Autodesk Inventor part; units mm, degrees
ref_plane "YZ Plane" through (0, 0, 0) normal (1, 0, 0) x (0, 1, 0)
ref_plane "XZ Plane" through (0, 0, 0) normal (0, 1, 0) x (-1, 0, 0)
ref_plane "XY Plane" through (0, 0, 0) normal (0, 0, 1) x (1, 0, 0)
sketch "Sketch1" plane through (0, 0, 0) normal (0, 1, 0) x (-1, 0, 0)
  circle A0 centre (0, 0) radius 15.875
  dimension "d7" = 31.75
extrude "Extrusion1" add sketch "Sketch1" along normal mid plane 159.2
sketch "Sketch2" plane through (0, 79.6, 0) normal (0, 1, 0) x (1, 0, 0)
  circle A0 centre (0, 0) radius 12.7
  circle A1 centre (0, 0) radius 15.875
  circle A2 centre (0, 0) radius 15.875
  dimension "d6" = 25.4
extrude "Extrusion2" cut sketch "Sketch2" against normal blind 54
fillet "Fillet1" radius 0.8 1 edges at (-12.7, 25.6, 0)
mirror "Mirror2" about plane through (0, -79.6, 0) normal (0, -1, 0) of "Extrusion2", "Extrusion1", "Fillet1"
properties part number "Eje Biela"
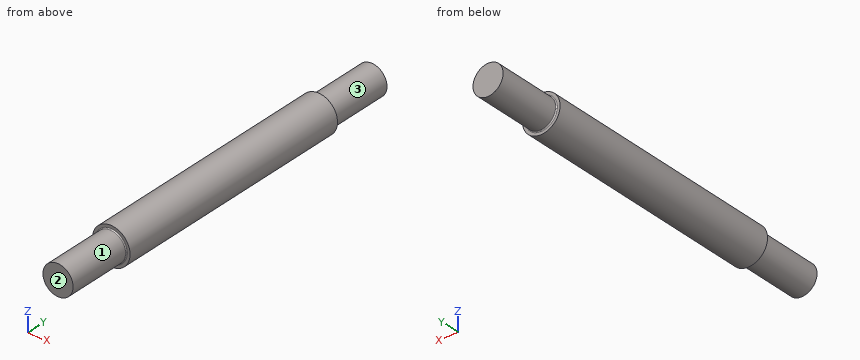
Build history of the part. All positions in model axes, mm. Face numbers are marked on the shaded views. A direction names the side the tool comes from. Give positions to 0.01 mm unless a question says otherwise; leave off trailing zeros. Write each loop counter-clockwise with the first axis right and the second up, starting at its lowest first coordinate (ties: lowest second). Pieces come first, ordered by that corner, then holes. Notation, with made-up numbers: (-17.75, 25) - (8.25, 25) arc R27 ccw to (8.25, 61) - close; hole circle Ø6 at (33, 31.5). An arc over 180 degrees is marked (long way). Use one line per item in the form item = value. Start each with the question number.
1. Band-saw the part on A-A on x = 0. Write the cut outline in (y, z) (3 decimals), plus the area to 3 significant figures.
2. Band-saw the part on C-C on y = -198.5. Write the cut outline in (x, z).
3. Band-saw the part on D-D on y = -149. Write the cut outline in (x, z) (3 decimals).
4. 3-axis set-ups, long thin cutter, end or side, ignore diameter. For the marked faces 1, 2 and 3: which of +Z, -Z, +X, -X, +Y, -Y reach the whole face in a straight line?
5. Probe line 1 (Z direction, x = -1, y = -197); line 2 (Y direction, x = -14, z = -5); line 3 (X direction, y = -84.5, z = 11). List the from-to ranges inside material, lowest first. Write a range as [from, to].
6. Band-saw the part on B-B on z = 0. Write the cut outline in (x, y) (3 decimals).
7. Drop flat-ended pins along their axis: pin 1 Ø2 at (y, z) = (21, 6.5) entering from +X; pin 2 Ø1 at (x, y) = (4.5, -129.5) entering from -Z; pin 3 Ø1 at (y, z) = (-1, -5) entering from -X. Give the stop position or say it passes through.
Conclusion:
q1.outline = (-238.8, -12.7) - (-185.6, -12.7) arc R0.8 cw to (-184.8, -13.5) - (-184.8, -15.875) - (25.6, -15.875) - (25.6, -13.5) arc R0.8 cw to (26.4, -12.7) - (79.6, -12.7) - (79.6, 12.7) - (26.4, 12.7) arc R0.8 cw to (25.6, 13.5) - (25.6, 15.875) - (-184.8, 15.875) - (-184.8, 13.5) arc R0.8 cw to (-185.6, 12.7) - (-238.8, 12.7) - close
q1.area = 9,420 mm²
q2.outline = circle Ø25.4 at (0, 0)
q3.outline = circle Ø31.75 at (0, 0)
q4.face_1 = -Y
q4.face_2 = +Z, -Z, +X, -X, -Y
q4.face_3 = +Y
q5.line_1 = [-12.66, 12.66]
q5.line_2 = [-184.8, 25.6]
q5.line_3 = [-11.45, 11.45]
q6.outline = (-15.875, -184.8) - (-13.5, -184.8) arc R0.8 cw to (-12.7, -185.6) - (-12.7, -238.8) - (12.7, -238.8) - (12.7, -185.6) arc R0.8 cw to (13.5, -184.8) - (15.875, -184.8) - (15.875, 25.6) - (13.5, 25.6) arc R0.8 cw to (12.7, 26.4) - (12.7, 79.6) - (-12.7, 79.6) - (-12.7, 26.4) arc R0.8 cw to (-13.5, 25.6) - (-15.875, 25.6) - close
q7.pin_1 = 14.89
q7.pin_2 = -15.36
q7.pin_3 = -15.22
